from build123d import *

# Parameters (mm, degrees)
SKETCH1_W           = 94
SKETCH1_H           = 85
BOSS_EXTRUDE1_DEPTH = 30
SKETCH2_W           = 35
SKETCH2_H           = 81
SKETCH2_W_2         = 25
SKETCH2_W_3         = 26
SKETCH2_H_2         = 33
SKETCH2_H_3         = 44
CUT_EXTRUDE1_DEPTH  = 28
SKETCH3_R           = 0.5
CUT_EXTRUDE2_DEPTH  = 28
SKETCH4_W           = 8
SKETCH4_H           = 11.916957973
CUT_EXTRUDE3_DEPTH  = 1
SKETCH5_R           = 4
CUT_EXTRUDE4_DEPTH  = 2
SKETCH6_W           = 5
SKETCH6_H           = 5
BOSS_EXTRUDE3_DEPTH = 28
SKETCH7_R           = 1.25
CUT_EXTRUDE5_DEPTH  = 20
FILLET1_R           = 1
SKETCH9_W           = 5
SKETCH9_H           = 33
BOSS_EXTRUDE4_DEPTH = 7
SKETCH10_W          = 5
SKETCH10_H          = 5
CUT_EXTRUDE7_DEPTH  = 39
FILLET3_R           = 2


with BuildPart() as part:
    # Sketch1 → Boss-Extrude1 (new body)
    with BuildSketch(Plane(origin=(0, 0, 0), x_dir=(1, 0, 0), z_dir=(0, 1, 0))):
        Rectangle(SKETCH1_W, SKETCH1_H)
    extrude(amount=BOSS_EXTRUDE1_DEPTH)

    # Sketch2 → Cut-Extrude1 (cut)
    with BuildSketch(Plane(origin=(0, 30, 0), x_dir=(1, 0, 0), z_dir=(0, 1, 0))):
        with Locations((-27.5, 0)):
            Rectangle(SKETCH2_W, SKETCH2_H)
        with Locations((4.5, 0)):
            Rectangle(SKETCH2_W_2, SKETCH2_H)
        with Locations((32, -24)):
            Rectangle(SKETCH2_W_3, SKETCH2_H_2)
        with Locations((32, 18.5)):
            Rectangle(SKETCH2_W_3, SKETCH2_H_3)
    extrude(amount=-CUT_EXTRUDE1_DEPTH, mode=Mode.SUBTRACT)

    # Sketch3 → Cut-Extrude2 (cut)
    with BuildSketch(Plane(origin=(0, 2, 0), x_dir=(1, 0, 0), z_dir=(0, 1, 0))):
        with Locations(Location((-30, -32.583042027, 0), (0, 0, 270))):
            Circle(SKETCH3_R)
        with Locations(Location((-26, -32.583042027, 0), (0, 0, 270))):
            Circle(SKETCH3_R)
    extrude(amount=-CUT_EXTRUDE2_DEPTH, mode=Mode.SUBTRACT)

    # Sketch4 → Cut-Extrude3 (cut)
    with BuildSketch(Plane(origin=(0, 0, 0), x_dir=(-1, 0, 0), z_dir=(0, -1, 0))):
        with Locations((28, -36.541521014)):
            Rectangle(SKETCH4_W, SKETCH4_H)
    extrude(amount=-CUT_EXTRUDE3_DEPTH, mode=Mode.SUBTRACT)

    # Sketch5 → Cut-Extrude4 (cut)
    with BuildSketch(Plane(origin=(19, 0, 0), x_dir=(0, 0, -1), z_dir=(1, 0, 0))):
        with Locations((18.5, 15)):
            Circle(SKETCH5_R)
    extrude(amount=-CUT_EXTRUDE4_DEPTH, mode=Mode.SUBTRACT)

    # Sketch6 → Boss-Extrude3 (add)
    with BuildSketch(Plane(origin=(0, 2, 0), x_dir=(1, 0, 0), z_dir=(0, 1, 0))):
        with Locations((42.5, 38)):
            Rectangle(SKETCH6_W, SKETCH6_H)
        with Locations((42.5, -1)):
            Rectangle(SKETCH6_W, SKETCH6_H)
    extrude(amount=BOSS_EXTRUDE3_DEPTH)

    # Sketch7 → Cut-Extrude5 (cut)
    with BuildSketch(Plane(origin=(0, 30, 0), x_dir=(1, 0, 0), z_dir=(0, 1, 0))):
        with Locations(Location((42.5, 38, 0), (0, 0, 270))):
            Circle(SKETCH7_R)
        with Locations(Location((42.5, -1, 0), (0, 0, 270))):
            Circle(SKETCH7_R)
    extrude(amount=-CUT_EXTRUDE5_DEPTH, mode=Mode.SUBTRACT)

    # Fillet1
    fillet1_edges = [part.edges().sort_by_distance(p)[0] for p in [
        (0, 30, 42.5),
        (47, 15, 42.5),
    ]]
    fillet(fillet1_edges, radius=FILLET1_R)

    # Sketch9 → Boss-Extrude4 (add)
    with BuildSketch(Plane(origin=(0, 2, 0), x_dir=(1, 0, 0), z_dir=(0, 1, 0))):
        with Locations((21.5, -24)):
            Rectangle(SKETCH9_W, SKETCH9_H)
    extrude(amount=BOSS_EXTRUDE4_DEPTH)

    # Sketch10 → Cut-Extrude7 (cut)
    with BuildSketch(Plane.XY.offset(42.5)):
        with Locations((20.5, 4.5)):
            Rectangle(SKETCH10_W, SKETCH10_H)
    extrude(amount=-CUT_EXTRUDE7_DEPTH, mode=Mode.SUBTRACT)

    # Fillet3
    fillet3_edges = [part.edges().sort_by_distance(p)[0] for p in [
        (24, 9, 24),
    ]]
    fillet(fillet3_edges, radius=FILLET3_R)


solid = part.part
Can you work these out from the model? Positions are in its coordinate system, mm. A direction names the side the tool comes from. Give positions to 0.01 mm unless a question says otherwise; leave off trailing zeros. Loops run counter-clockwise (first coordinate to the right, second up) from the corner with the lowest first, then second, coordinate; pieces in that order, holes last. Notation, with made-up numbers: (31, -9.75) -> (42, -9.75) arc R9 ccw to (42, -4.75) -> close; hole circle Ø4 at (40.5, 44.5). An arc over 180 degrees is marked (long way). Return JSON: item names as keys, results as strings.
Q1. I want a section at C-C, the plane y = 15. Count the separate pieces of the cut face and the enclosed holes in it, then the cut area to 3 significant figures.
Checks:
{"separate pieces": "1", "enclosed holes": "5", "area": "1,150 mm2"}
Q2. I want a section at D-D, the plane y = 27.5. List the corners of the cut face in (x, z) for me, then the cut area to 3 significant figures.
Checks:
{"outline": "(-47, -42.5) -> (47, -42.5) -> (47, 41.5) arc R1 ccw to (46, 42.5) -> (-47, 42.5) -> close; hole (-45, -40.5) -> (-10, -40.5) -> (-10, 40.5) -> (-45, 40.5) -> close; hole (-8, -40.5) -> (17, -40.5) -> (17, 40.5) -> (-8, 40.5) -> close; hole (19, -40.5) -> (40, -40.5) -> (40, -35.5) -> (45, -35.5) -> (45, -1.5) -> (40, -1.5) -> (40, 3.5) -> (19, 3.5) -> close; hole (19, 7.5) -> (45, 7.5) -> (45, 40.5) -> (19, 40.5) -> close; hole circle Ø2.5 at (42.5, -38); hole circle Ø2.5 at (42.5, 1)", "area": "1,170 mm2"}
Q3. We'd pull the mould along Z, two halves only. Please class faces 1 (the face through (34, 2, 24)), 2 (the face through (17.2, 30, -6.9)): released by +Z, released by -Z, zero draft, split by the parting line, or undercut.
Checks:
{"face 1": "undercut", "face 2": "zero draft"}
Q4. For pin 1 Ø1 at (x, z) = (-21.5, 33.5) entering from +Y; pin 2 Ø2.5 at (x, z) = (-29, 37) entering from -Y, each with a flat end and sliding along its axis, tell me the tip position at first contact or that it passes through.
Checks:
{"pin 1": "stops at y = 2", "pin 2": "stops at y = 1"}
Q5. I need wall thicknesses on probe 1 along X at (y, z) = (11.5, 21); probe 2 along X at (y, z) = (6.5, 35.5); probe 3 along X at (y, z) = (3, -37.5). Which ranges of each line are inside material? Lowest first, please.
Checks:
{"probe 1": "x = -47 to -45, -10 to -8, 17 to 19, 45 to 47", "probe 2": "x = -47 to -45, -10 to -8, 17 to 18, 23 to 24, 45 to 47", "probe 3": "x = -47 to -45, -10 to -8, 17 to 19, 40 to 47"}
Q6. I want a section at B-B, the plane x = 4.5. List the corners of the cut face in (y, z) for me.
Checks:
{"outline": "(0, -42.5) -> (30, -42.5) -> (30, -40.5) -> (2, -40.5) -> (2, 40.5) -> (30, 40.5) -> (30, 41.5) arc R1 ccw to (29, 42.5) -> (0, 42.5) -> close"}
Q7. I want a section at A-A, the plane z = -38. List the corners of the cut face in (x, y) for me, then the cut area to 3 significant figures.
Checks:
{"outline": "(-47, 0) -> (47, 0) -> (47, 30) -> (43.75, 30) -> (43.75, 10) -> (41.25, 10) -> (41.25, 30) -> (40, 30) -> (40, 2) -> (19, 2) -> (19, 30) -> (17, 30) -> (17, 2) -> (-8, 2) -> (-8, 30) -> (-10, 30) -> (-10, 2) -> (-45, 2) -> (-45, 30) -> (-47, 30) -> close", "area": "502 mm2"}
Q8. On a 3-axis mill with a long thin cutter (end or side, diameter ignored), from which of +Z, -Z, +X, -X, +Y, -Y can I reach the whole of each face in a straight line? I mean faces 3 (the face through (40, 16, -38)), 4 (the face through (28, 2, -9)), 5 (the face through (23, 4, 23)). Say none if no direction works.
Checks:
{"face 3": "+Y", "face 4": "none", "face 5": "+Z"}
